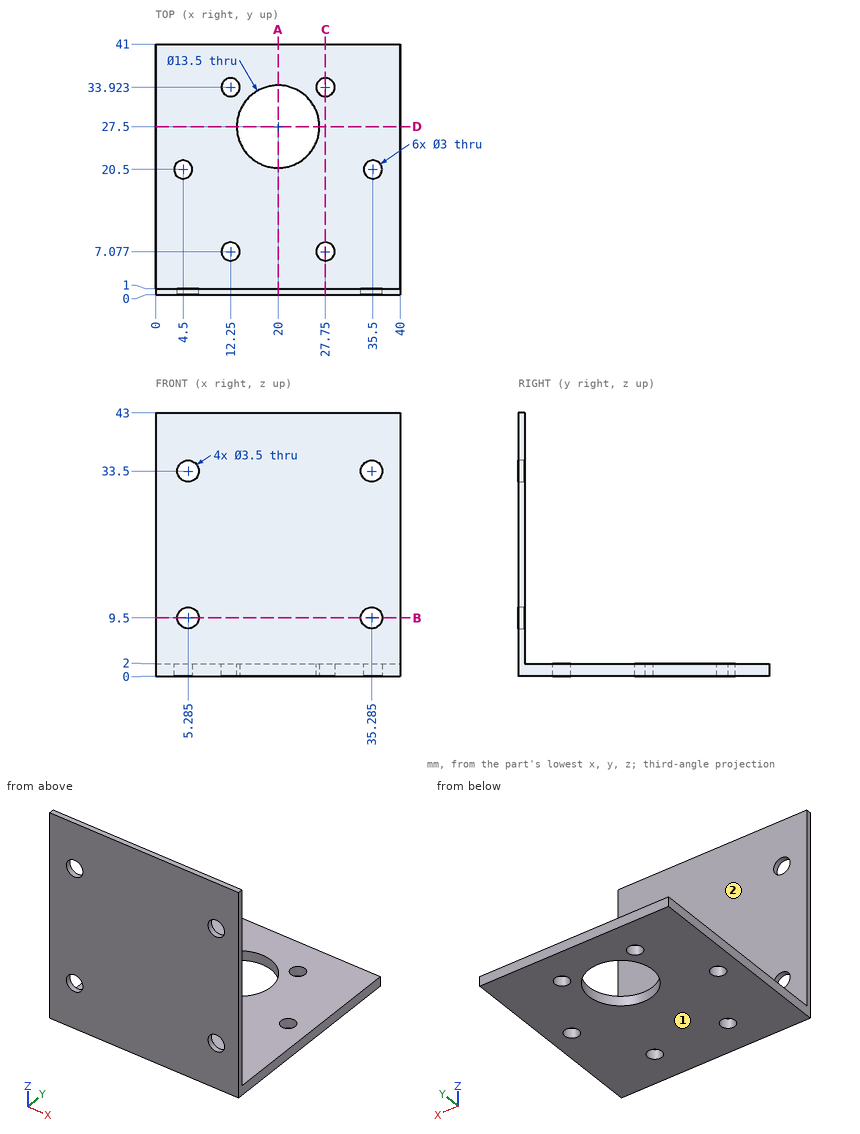
Study the drawing (mm; zero at the part's minimum x, y, z) and answer. A direction names the side the tool comes from. Give positions to 0.01 mm unless a question says otherwise; leave off trailing zeros. Write each loop counter-clockwise with the first axis right and the second up, starting at its lowest first coordinate (ties: lowest second). Pieces come first, ordered by that corner, then holes.
Item 1: Which of the six approach directions +Z, -Z, +X, -X, +Y, -Y give full straight-line access (tool end or side, diameter ignored) to the marked faces 1 and 2?
Item 2: Section A-A, the plane x = 20 is taken. Write down the section's boundary in (y, z).
Item 3: Find the intervals of material crossed by line 1 along X through (y, z) = (0.4, 33.5) (1 decimal); line 2 along Y through (x, z) = (27, 1) (1 decimal); line 3 along Y through (x, z) = (11, 34.5), in increasing order.
Item 4: Flat-ended cylindrical pins translate along their axes: P1, Ø5.5, axis at x = 5.28, z = 9.5, coming from the +Y side; P2, Ø3.5, axis at x = 35.5, y = 20.5, coming from the +Z side. Find the tip coordinate at first contact, or state that the pin passes through.
Item 5: Section C-C, the plane x = 27.75 is taken. Write down the section's boundary in (y, z).
Item 6: Section B-B, the plane z = 9.5 is taken. Write down the section's boundary in (x, y) (1 decimal).
Item 7: Section D-D, the plane y = 27.5 is taken. Write down the section's boundary in (x, z).
Completed:
1. face 1: -Z, +X, -X, +Y, -Y
1. face 2: +Z, +X, -X, +Y
2. outline: (0, 0) - (20.75, 0) - (20.75, 2) - (1, 2) - (1, 43) - (0, 43) - close; (34.25, 0) - (41, 0) - (41, 2) - (34.25, 2) - close
3. line 1: x = 0 to 3.5, 7 to 33.5, 37 to 40
3. line 2: y = 0 to 5.8, 8.4 to 32.6, 35.2 to 41
3. line 3: y = 0 to 1
4. P1: stops at y = 1
4. P2: stops at z = 2
5. outline: (0, 0) - (5.58, 0) - (5.58, 2) - (1, 2) - (1, 43) - (0, 43) - close; (8.58, 0) - (32.42, 0) - (32.42, 2) - (8.58, 2) - close; (35.42, 0) - (41, 0) - (41, 2) - (35.42, 2) - close
6. outline: (0, 0) - (3.5, 0) - (3.5, 1) - (0, 1) - close; (7, 0) - (33.5, 0) - (33.5, 1) - (7, 1) - close; (37, 0) - (40, 0) - (40, 1) - (37, 1) - close
7. outline: (0, 0) - (13.25, 0) - (13.25, 2) - (0, 2) - close; (26.75, 0) - (40, 0) - (40, 2) - (26.75, 2) - close
